Source: CAD feature listing. Evaluate the final solid. Frame: model axes, mm. Face numbers are marked on the shaded views. A direction names the side the tool comes from. Give positions to 0.01 mm unless a question says otherwise; leave off trailing zeros. Order: outer loops, then holes, each group sorted by start corner. A loop starts at its lowest first (then second) coordinate and runs counter-clockwise, first axis right, second up. Notation, with made-up numbers: M 31.25,52.25 L 74.25,52.25 A13 cw 74.25,60.25 Z; hole C -6,-30.5 d5. An arc over 180 degrees is marked long. Use CSV: the item, a comma, the result in double quotes. Start each with the question number.
Item 1: Access query for the marked faces 1, 2 and 3. Directions: +Z, -Z, +X, -X, +Y, -Y. A direction counts if a zero-diameter tool reaches every point of the face in a straight line with its end or side. Return the directions, or none.
Item 2: Section query D-D on y = 7.25. Return loops of the section in (x, z).
Item 3: Ray query, probe 1 along X at (y, z) = (-8.25, 5.25); probe 2 along Y at (x, z) = (0.5, -2.5); probe 3 along X at (y, z) = (5.5, -5.5). Return the intervals inside material, ascending. Write a range as from..to.
Item 4: Section query B-B on x = -4.5. Return loops of the section in (y, z), and give its area (3 significant figures).
Item 5: Section query A-A on y = 0. Return loops of the section in (x, z), and give its area (3 significant figures).
Item 6: Section query C-C on z = 5. Return loops of the section in (x, y).
Item 7: First-contact query: pin 1 (7 mm diameter, centred on y = 3.5, z = -4.5, fed in from +X); pin 2 (1.9 mm diameter, centred on x = -13.75, y = 0, fed in from -Z); pin 3 (1.6 mm diameter, centred on x = -2.5, z = 3, fed in from -Y); pin 4 (3 mm diameter, centred on x = -10, y = -3, fed in from +Z). Flat tips, straight axial feed; report the tip coordinate or a pass-through.
from build123d import *

# Parameters (mm, degrees)
SKETCH1_R           = 1.6
SKETCH1_W           = 15.8
SKETCH1_H           = 13.25
BOSS_EXTRUDE1_DEPTH = 6.8
BOSS_EXTRUDE4_DEPTH = 6
SKETCH6_W           = 4
SKETCH6_H           = 4
BOSS_EXTRUDE6_DEPTH = 4
FILLET1_R           = 0.5


with BuildPart() as part:
    # Sketch1 → Boss-Extrude1 (new body)
    with BuildSketch(Plane.XY):
        with BuildLine():
            Line((-11, 4.75), (-11, 11))
            Line((-11, 11), (11, 11))
            Line((11, 11), (11, 4.75))
            Line((11, 4.75), (13.75, 4.75))
            ThreePointArc((13.75, 4.75), (18.5, 0), (13.75, -4.75))
            Line((13.75, -4.75), (11, -4.75))
            Line((11, -4.75), (11, -11))
            Line((11, -11), (22, -11))
            Line((22, -11), (22, 14.2))
            Line((22, 14.2), (-22, 14.2))
            Line((-22, 14.2), (-22, -11))
            Line((-22, -11), (-11, -11))
            Line((-11, -11), (-11, -4.75))
            Line((-11, -4.75), (-13.75, -4.75))
            ThreePointArc((-13.75, -4.75), (-18.5, 0), (-13.75, 4.75))
            Line((-13.75, 4.75), (-11, 4.75))
        make_face()
        with BuildLine():
            Line((13.75, -4.75), (11, -4.75))
            Line((11, -4.75), (11, -11))
            Line((11, -11), (-11, -11))
            Line((-11, -11), (-11, -4.75))
            Line((-11, -4.75), (-13.75, -4.75))
            ThreePointArc((-13.75, -4.75), (-18.5, 0), (-13.75, 4.75))
            Line((-13.75, 4.75), (-11, 4.75))
            Line((-11, 4.75), (-11, 11))
            Line((-11, 11), (11, 11))
            Line((11, 11), (11, 4.75))
            Line((11, 4.75), (13.75, 4.75))
            ThreePointArc((13.75, 4.75), (18.5, 0), (13.75, -4.75))
        make_face()
        with Locations((13.75, 0)):
            Circle(SKETCH1_R, mode=Mode.SUBTRACT)
        with Locations((-13.75, 0)):
            Circle(SKETCH1_R, mode=Mode.SUBTRACT)
        with Locations((0, 1.625)):
            Rectangle(SKETCH1_W, SKETCH1_H, mode=Mode.SUBTRACT)
    extrude(amount=-BOSS_EXTRUDE1_DEPTH)

    # Sketch1_3 → Boss-Extrude4 (add)
    with BuildSketch(Plane.XY):
        with BuildLine():
            Line((-11, 4.75), (-11, 11))
            Line((-11, 11), (11, 11))
            Line((11, 11), (11, 4.75))
            Line((11, 4.75), (13.75, 4.75))
            ThreePointArc((13.75, 4.75), (18.5, 0), (13.75, -4.75))
            Line((13.75, -4.75), (11, -4.75))
            Line((11, -4.75), (11, -11))
            Line((11, -11), (22, -11))
            Line((22, -11), (22, 14.2))
            Line((22, 14.2), (-22, 14.2))
            Line((-22, 14.2), (-22, -11))
            Line((-22, -11), (-11, -11))
            Line((-11, -11), (-11, -4.75))
            Line((-11, -4.75), (-13.75, -4.75))
            ThreePointArc((-13.75, -4.75), (-18.5, 0), (-13.75, 4.75))
            Line((-13.75, 4.75), (-11, 4.75))
        make_face()
    extrude(amount=BOSS_EXTRUDE4_DEPTH)

    # Sketch6 → Boss-Extrude6 (add)
    with BuildSketch(Plane(origin=(22, 0, 0), x_dir=(0, 0, -1), z_dir=(1, 0, 0))):
        with Locations((-1.2, -9)):
            Rectangle(SKETCH6_W, SKETCH6_H)
    extrude(amount=BOSS_EXTRUDE6_DEPTH)

    # Fillet1
    fillet1_edges = [part.edges().sort_by_distance(p)[0] for p in [
        (-7.9, 1.625, 0),
        (0, -11, -6.8),
        (0, -5, 0),
        (7.9, 1.625, 0),
        (0, 8.25, 0),
        (22, 1.6, -6.8),
        (22, -11, -3.8),
        (-22, -11, -0.4),
        (0, -11, 0),
        (18.5, 0, 6),
        (11, -4.75, 3),
        (16.5, -11, 6),
        (11, -11, 3),
        (22, 1.6, 6),
        (-22, 1.6, 6),
        (-16.5, -11, 6),
        (-11, -7.875, 6),
        (-11, -11, 3),
        (-12.375, -4.75, 6),
        (-11, -4.75, 3),
        (-18.5, 0, 6),
        (-11, 7.875, 6),
        (-11, 4.75, 3),
        (12.375, 4.75, 6),
        (11, 4.75, 3),
        (12.375, -4.75, 6),
        (11, -7.875, 6),
        (-12.375, 4.75, 6),
        (0, 11, 6),
        (11, 7.875, 6),
        (22, -11, 4.6),
        (22, -9, 3.2),
        (24, -7, 3.2),
        (24, -11, 3.2),
        (22, -9, -0.8),
        (24, -11, -0.8),
        (22, -7, 1.2),
        (24, -7, -0.8),
        (26, -9, 3.2),
        (26, -11, 1.2),
        (26, -9, -0.8),
        (26, -7, 1.2),
        (-22, 1.6, -6.8),
    ]]
    fillet(fillet1_edges, radius=FILLET1_R)


solid = part.part
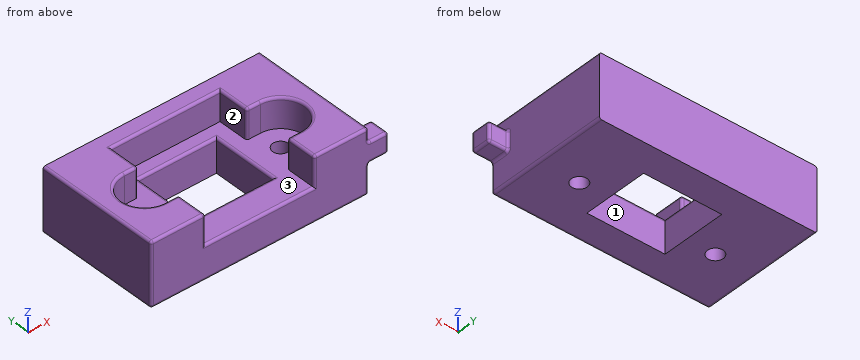
Verdict:
1,face 1,"+Z, -Z"
1,face 2,"+Z, -Y"
1,face 3,"+Z"
2,outline,"M -22,-6.3 A0.5 ccw -21.5,-6.8 L -7.9,-6.8 L -7.9,-0.5 A0.5 ccw -8.4,0 L -11,0 L -11,5.5 A0.5 ccw -11.5,6 L -21.5,6 A0.5 ccw -22,5.5 Z; M 7.9,-6.8 L 21.5,-6.8 A0.5 ccw 22,-6.3 L 22,5.5 A0.5 ccw 21.5,6 L 11.5,6 A0.5 ccw 11,5.5 L 11,0 L 8.4,0 A0.5 ccw 7.9,-0.5 Z"
3,probe 1,"-22..-11, 11..22"
3,probe 2,"-11..-5, 8.25..14.2"
3,probe 3,"-22..-7.9, 7.9..22"
4,outline,"M -11,-6.3 A0.5 ccw -10.5,-6.8 L -5,-6.8 L -5,-0.5 A0.5 ccw -5.5,0 L -10.5,0 A0.5 ccw -11,-0.5 Z; M 8.25,-6.8 L 14.2,-6.8 L 14.2,6 L 11.5,6 A0.5 ccw 11,5.5 L 11,0 L 8.75,0 A0.5 ccw 8.25,-0.5 Z"
4,area,"100 mm2"
5,outline,"M -22,-6.3 A0.5 ccw -21.5,-6.8 L -15.35,-6.8 L -15.35,0 L -18.5,0 L -18.5,5.5 A0.5 ccw -19,6 L -21.5,6 A0.5 ccw -22,5.5 Z; M -12.15,-6.8 L -7.9,-6.8 L -7.9,-0.5 A0.5 ccw -8.4,0 L -12.15,0 Z; M 7.9,-6.8 L 12.15,-6.8 L 12.15,0 L 8.4,0 A0.5 ccw 7.9,-0.5 Z; M 15.35,-6.8 L 21.5,-6.8 A0.5 ccw 22,-6.3 L 22,5.5 A0.5 ccw 21.5,6 L 19,6 A0.5 ccw 18.5,5.5 L 18.5,0 L 15.35,0 Z"
5,area,"190 mm2"
6,outline,"M -22,-10.5 A0.5 ccw -21.5,-11 L -11.5,-11 A0.5 ccw -11,-10.5 L -11,-5.25 A0.5 ccw -11.5,-4.75 L -13.75,-4.75 A4.75 cw -13.75,4.75 L -11.5,4.75 A0.5 ccw -11,5.25 L -11,11 L 11,11 L 11,5.25 A0.5 ccw 11.5,4.75 L 13.75,4.75 A4.75 cw 13.75,-4.75 L 11.5,-4.75 A0.5 ccw 11,-5.25 L 11,-10.5 A0.5 ccw 11.5,-11 L 21.5,-11 A0.5 ccw 22,-10.5 L 22,14.2 L -22,14.2 Z"
7,pin 1,"x = 22"
7,pin 2,"through"
7,pin 3,"y = 11"
7,pin 4,"z = 0"
